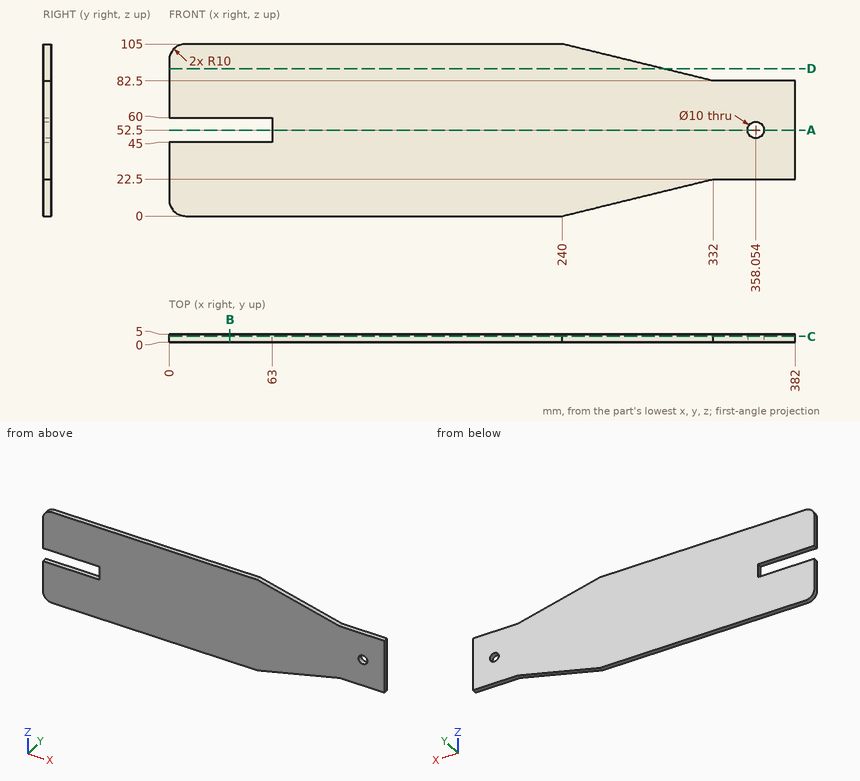
Drawing for the job (mm, zero at the part's lowest x, y, z). Round coordinates to 2 decimals unless told otherwise and drop trailing zeros. Loops run counter-clockwise (first coordinate to the right, second up) from the corner with the lowest first, then second, coordinate; pieces in that order, holes last. Notation, with made-up numbers: M -36.5,72 L -26.5,72 A26 cw -26.5,92 Z; hole C 81,-40 d9. An arc over 180 degrees is marked long. Use a Markdown table: item, result. Add a question column.
(1) Cut at C-C (y = 3.55). Give the cut face in (x, z).
(2) Cut at A-A (z = 52.5). Give the cut face in (x, y).
(3) Cut at D-D (z = 90). Give the cut face in (x, y).
(4) Flat gauge pin, fed straight in: pin 1 (1.5 mm diameter, centred on x = 362.5, y = 3.5, fed in from -Z). Where does the tip first touch, or does it go through?
(5) Drill centre lines: line 1 (Z direction, x = 16, y = 2.1); line 2 (Z direction, x = 349.5, y = 2.5); line 3 (X direction, y = 1.45, z = 50) (1 decimal). Where is each one in solid material? Low to high.
(6) Cut at B-B (x = 37). Give the cut face in (y, z).
Geometry says:
| question | item | result |
|---|---|---|
| 1 | outline | M 0,10 A10 ccw 10,0 L 240,0 L 332,22.5 L 382,22.5 L 382,82.5 L 332,82.5 L 240,105 L 10,105 A10 ccw 0,95 L 0,60 L 63,60 L 63,45 L 0,45 Z; hole C 358.05,52.5 d10 |
| 2 | outline | M 63,0 L 353.05,0 L 353.05,5 L 63,5 Z; M 363.05,0 L 382,0 L 382,5 L 363.05,5 Z |
| 3 | outline | M 0,0 L 301.33,0 L 301.33,5 L 0,5 Z |
| 4 | pin 1 | stops at z = 22.5 |
| 5 | line 1 | z = 0 to 45, 60 to 105 |
| 5 | line 2 | z = 22.5 to 82.5 |
| 5 | line 3 | x = 63 to 353.7, 362.4 to 382 |
| 6 | outline | M 0,0 L 5,0 L 5,45 L 0,45 Z; M 0,60 L 5,60 L 5,105 L 0,105 Z |
